Could you check a few things on this model? Use its own coordinates, in mm. Coordinates: 2 decimals unless noted, no trailing zeros. One line per question, with ' | ' between items. Start each with the question number.
1. We'd pull the mould along X, two halves only. Please class faces 1 (the flat face through (15, 27, 1.6)), 2 (the cylindrical face through (26.74, 2.58, 0.79)), 3 (the flat face through (0, 27, 1)): pulls with the +X half, pulls with the -X half, needs draft (parallel to the pull), parting line crosses it, or undercut.
2. I want a section at A-A, the plane z = 1.05. Count the separate pieces of the cut face and the enclosed holes in it, then the cut area to 3 significant figures.
3. Please list where these lines run through material, in increasing order: L1, parallel to X at y = 47, z = 0.45; L2, parallel to Y at x = 25, z = 0.2; L3, parallel to Y at x = 3.75, z = 1.2. Write a range as [from, to].
4. I'm going to push a flat-ended pin straight in: P1, Ø2.5, axis at x = 26, y = 50, coming from the +Z side. Where does the tip first touch, or does it pass through?
from build123d import *

# Parameters (mm, degrees)
MODEL_W            = 30
MODEL_H            = 54
MODEL_R            = 0.5
MODEL_R_2          = 0.65
MODEL_R_3          = 0.45
MODEL_R_4          = 0.75
MODEL_R_5          = 1.8
MODEL_R_6          = 0.6
MODEL_R_7          = 1.55
MODEL_R_8          = 0.35
MODEL_R_9          = 1
MODEL_R_10         = 1.6
MODEL_R_11         = 0.2
BOSS_EXTRU_1_DEPTH = 1.6


with BuildPart() as part:
    # Model → Boss.-Extru.1 (new body)
    with BuildSketch(Plane.XY):
        with Locations((15, 27)):
            Rectangle(MODEL_W, MODEL_H)
        with Locations((5.79882, 28.75026)):
            Circle(MODEL_R, mode=Mode.SUBTRACT)
        with Locations((6.88975, 18.04924)):
            Circle(MODEL_R_2, mode=Mode.SUBTRACT)
        with Locations((10.60069, 27.0002)):
            Circle(MODEL_R_2, mode=Mode.SUBTRACT)
        with Locations((1.70053, 30.8991)):
            Circle(MODEL_R_3, mode=Mode.SUBTRACT)
        with Locations((19.00047, 41.40074)):
            Circle(MODEL_R_4, mode=Mode.SUBTRACT)
        with Locations((5.79882, 25.25026)):
            Circle(MODEL_R, mode=Mode.SUBTRACT)
        with Locations((7.89882, 27.00026)):
            Circle(MODEL_R, mode=Mode.SUBTRACT)
        with Locations((3.49882, 27.00026)):
            Circle(MODEL_R, mode=Mode.SUBTRACT)
        with Locations((1.49882, 27.00026)):
            Circle(MODEL_R, mode=Mode.SUBTRACT)
        with Locations((10.60069, 29.5402)):
            Circle(MODEL_R_2, mode=Mode.SUBTRACT)
        with Locations((14.99997, 20.69973)):
            Circle(MODEL_R_4, mode=Mode.SUBTRACT)
        with Locations((14.99997, 43.29973)):
            Circle(MODEL_R_4, mode=Mode.SUBTRACT)
        with Locations((19.00047, 46.40074)):
            Circle(MODEL_R_4, mode=Mode.SUBTRACT)
        with Locations((11.50047, 36.40074)):
            Circle(MODEL_R_4, mode=Mode.SUBTRACT)
        with Locations((11.50047, 41.40074)):
            Circle(MODEL_R_4, mode=Mode.SUBTRACT)
        with Locations((11.50047, 46.40074)):
            Circle(MODEL_R_4, mode=Mode.SUBTRACT)
        with Locations((27.49931, 39.20108)):
            Circle(MODEL_R_3, mode=Mode.SUBTRACT)
        with Locations((27.49931, 34.20108)):
            Circle(MODEL_R_3, mode=Mode.SUBTRACT)
        with Locations((27.50058, 27.00058)):
            Circle(MODEL_R_5, mode=Mode.SUBTRACT)
        with Locations((5.99948, 39.80942)):
            Circle(MODEL_R_6, mode=Mode.SUBTRACT)
        with Locations((24.33058, 24.50058)):
            Circle(MODEL_R_7, mode=Mode.SUBTRACT)
        with Locations((27.50058, 19.80058)):
            Circle(MODEL_R, mode=Mode.SUBTRACT)
        with Locations((7.78891, 9.4996)):
            Circle(MODEL_R_8, mode=Mode.SUBTRACT)
        with Locations((2.70891, 9.4996)):
            Circle(MODEL_R_8, mode=Mode.SUBTRACT)
        with Locations((15.67058, 24.50058)):
            Circle(MODEL_R_7, mode=Mode.SUBTRACT)
        with Locations((27.50058, 9.79932)):
            Circle(MODEL_R, mode=Mode.SUBTRACT)
        with Locations((6.88975, 15.50924)):
            Circle(MODEL_R_2, mode=Mode.SUBTRACT)
        with Locations((20.00058, 32.00058)):
            Circle(MODEL_R_7, mode=Mode.SUBTRACT)
        with Locations((12.31711, 50.41646)):
            Circle(MODEL_R_3, mode=Mode.SUBTRACT)
        with Locations((21.41711, 50.41646)):
            Circle(MODEL_R_9, mode=Mode.SUBTRACT)
        with Locations((8.41711, 50.41646)):
            Circle(MODEL_R_9, mode=Mode.SUBTRACT)
        with Locations((1.70053, 12.19962)):
            Circle(MODEL_R_3, mode=Mode.SUBTRACT)
        with Locations((20.49907, 11.303)):
            Circle(MODEL_R_10, mode=Mode.SUBTRACT)
        with Locations((14.9987, 14.50213)):
            Circle(MODEL_R_10, mode=Mode.SUBTRACT)
        with Locations((9.4996, 4.20243)):
            Circle(MODEL_R_10, mode=Mode.SUBTRACT)
        with Locations((6.88975, 20.58924)):
            Circle(MODEL_R_2, mode=Mode.SUBTRACT)
        with Locations((10.60069, 24.4602)):
            Circle(MODEL_R_2, mode=Mode.SUBTRACT)
        with Locations((1.70053, 23.20036)):
            Circle(MODEL_R_3, mode=Mode.SUBTRACT)
        with Locations((27.50058, 14.80058)):
            Circle(MODEL_R, mode=Mode.SUBTRACT)
        with Locations((20.73656, 27.4828)):
            Circle(MODEL_R_11, mode=Mode.SUBTRACT)
        with Locations((8.89508, 37.16528)):
            Circle(MODEL_R_11, mode=Mode.SUBTRACT)
        with Locations((6.00329, 45.26788)):
            Circle(MODEL_R_3, mode=Mode.SUBTRACT)
        with Locations((1.70053, 41.89984)):
            Circle(MODEL_R_3, mode=Mode.SUBTRACT)
        with Locations((19.00047, 36.40074)):
            Circle(MODEL_R_4, mode=Mode.SUBTRACT)
        with Locations((27.49931, 44.20108)):
            Circle(MODEL_R_3, mode=Mode.SUBTRACT)
        with Locations((5.99948, 32.18942)):
            Circle(MODEL_R_6, mode=Mode.SUBTRACT)
        with Locations((19.00047, 21.3995)):
            Circle(MODEL_R_4, mode=Mode.SUBTRACT)
        with Locations((5.24891, 9.4996)):
            Circle(MODEL_R_8, mode=Mode.SUBTRACT)
        with Locations((21.49983, 15.40002)):
            Circle(MODEL_R_3, mode=Mode.SUBTRACT)
        with Locations((6.00329, 42.72788)):
            Circle(MODEL_R_3, mode=Mode.SUBTRACT)
        with Locations((17.51711, 50.41646)):
            Circle(MODEL_R_3, mode=Mode.SUBTRACT)
        with Locations((3.89763, 34.88182)):
            Circle(MODEL_R, mode=Mode.SUBTRACT)
        with Locations((7.99592, 34.55416)):
            Circle(MODEL_R, mode=Mode.SUBTRACT)
        with Locations((18.50009, 15.40002)):
            Circle(MODEL_R_3, mode=Mode.SUBTRACT)
        with Locations((11.49985, 21.3995)):
            Circle(MODEL_R_4, mode=Mode.SUBTRACT)
        with Locations((4, 50)):
            Circle(MODEL_R_10, mode=Mode.SUBTRACT)
        with Locations(Location((26, 50, 0), (0, 0, 180))):
            Circle(MODEL_R_10, mode=Mode.SUBTRACT)
        with Locations((26, 4)):
            Circle(MODEL_R_10, mode=Mode.SUBTRACT)
        with Locations(Location((4, 4, 0), (0, 0, 180))):
            Circle(MODEL_R_10, mode=Mode.SUBTRACT)
        with Locations((12.40028, 3.50012)):
            Circle(MODEL_R, mode=Mode.SUBTRACT)
        with Locations((15.00028, 3.50012)):
            Circle(MODEL_R_9, mode=Mode.SUBTRACT)
        with Locations((17.60028, 3.50012)):
            Circle(MODEL_R, mode=Mode.SUBTRACT)
    extrude(amount=BOSS_EXTRU_1_DEPTH)


solid = part.part
Results are:
1) face 1: needs draft | face 2: undercut | face 3: pulls with the -X half
2) separate pieces: 1 | enclosed holes: 62 | area: 1,470 mm2
3) L1: x = [0, 11.05], [11.95, 18.55], [19.45, 30] | L2: y = [0, 2.75], [5.25, 23.1], [25.9, 48.75], [51.25, 54] | L3: y = [0, 2.42], [5.58, 26.57], [27.43, 34.4], [35.36, 48.42], [51.58, 54]
4) P1: passes through
